Can you work these out from the drawing? Everything is in mm from the part's minimum corner. Round coordinates to 2 decimals unless told otherwise and drop trailing zeros. Write each loop counter-clockwise with the first axis right and the second up, starting at its lowest first coordinate (ties: lowest second). Pieces come first, ordered by that corner, then holes. Notation, with made-up numbers: M 14.25,63.5 L 36.25,63.5 A27 cw 36.25,90.5 Z; hole C 26.25,3.25 d4. An arc over 180 degrees is marked long. Use one line per item in the form item = value. Start each with the question number.
Q1. We'd pull the mould along X, two halves only. Please class the marked faces 1, 2, 3 and 4: +X half, -X half, draft (parallel to the pull), parting line (faces both ways), or undercut.
Q2. I want a section at C-C on x = 76.2. List the corners of the cut face in (y, z) for me, and give its area (3 significant figures).
Q3. I want a section at A-A on y = 36.5. List the corners of the cut face in (x, z) for me, and give its area (3 significant figures).
Q4. I'm going to push flat-ended pins straight in: pin 1 Ø8 at (y, z) = (35, 68) entering from +X; pin 2 Ø23 at (x, z) = (76.2, 50.8) entering from -Y; pin 3 Ø1.5 at (x, y) = (117, 6.5) entering from +Z; pin 4 Ø2 at (y, z) = (7, 42.5) entering from -X (3 decimals). Where does each tip first touch, or does it pass through?
Q5. I want a section at B-B on z = 50.8. List the corners of the cut face in (x, y) for me, and give its area (3 significant figures).
Q6. I need wall thicknesses on line 1 along Z through (x, y) = (76, 14); line 2 along X through (y, z) = (30, 50); line 3 along X through (y, z) = (36, 35.5) (3 decimals). Which ranges of each line are inside material? Lowest first, please. Write a range as from..to.
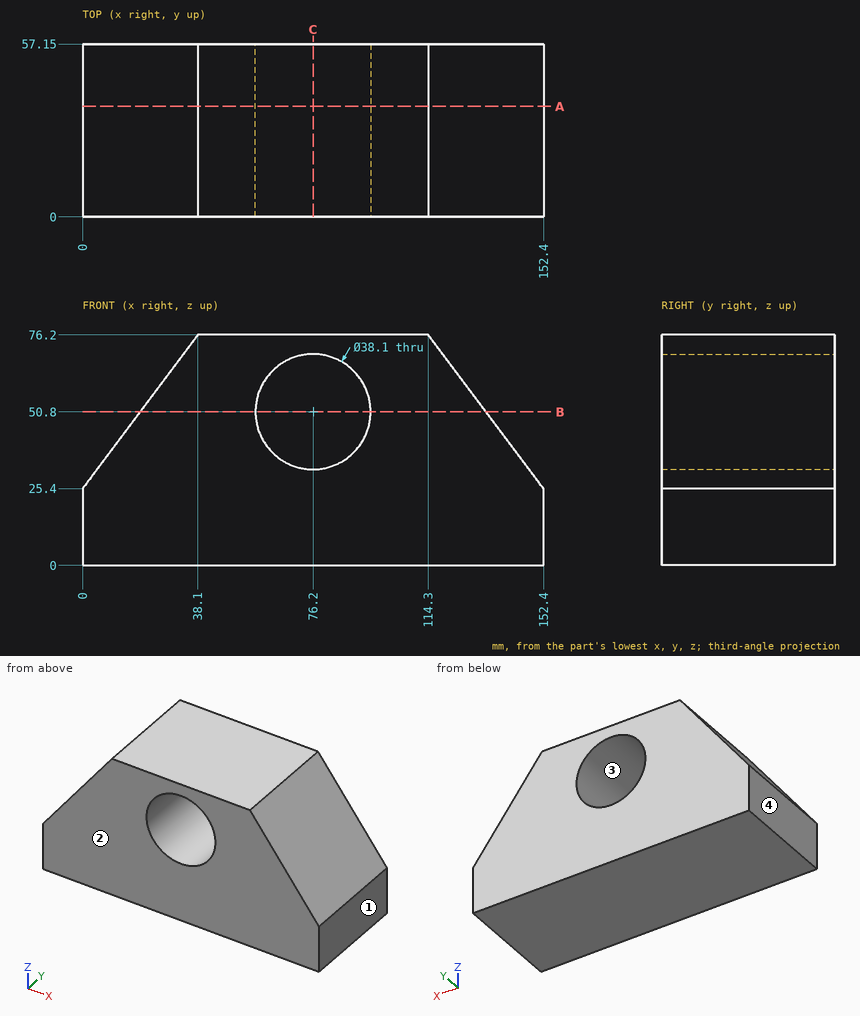
Reported:
q1.face_1 = +X half
q1.face_2 = draft
q1.face_3 = undercut
q1.face_4 = -X half
q2.outline = M 0,0 L 57.15,0 L 57.15,31.75 L 0,31.75 Z; M 0,69.85 L 57.15,69.85 L 57.15,76.2 L 0,76.2 Z
q2.area = 2,180 mm^2
q3.outline = M 0,0 L 152.4,0 L 152.4,25.4 L 114.3,76.2 L 38.1,76.2 L 0,25.4 Z; hole C 76.2,50.8 d38.1
q3.area = 8,540 mm^2
q4.pin_1 = 123.45
q4.pin_2 = through
q4.pin_3 = 73.6
q4.pin_4 = 12.075
q5.outline = M 19.05,0 L 57.15,0 L 57.15,57.15 L 19.05,57.15 Z; M 95.25,0 L 133.35,0 L 133.35,57.15 L 95.25,57.15 Z
q5.area = 4,350 mm^2
q6.line_1 = 0..31.75, 69.85..76.2
q6.line_2 = 18.45..57.17, 95.23..133.95
q6.line_3 = 7.575..64.85, 87.55..144.825
